from build123d import *

# Parameters (mm, degrees)
ESBO_O1_R                = 27.71344859
ESBO_O1_R_2              = 19.642943244
ESBO_O1_R_3              = 19
ESBO_O1_R_4              = 13.503376128
ESBO_O1_R_5              = 12.848056377
ESBO_O1_R_6              = 13.183675058
ESBO_O1_R_7              = 19.84940304
ESBO_O1_R_8              = 26.715530758
RESSALTO_EXTRUS_O1_DEPTH = 25


with BuildPart() as part:
    # Esboço1 → Ressalto-extrusão1 (new body)
    with BuildSketch(Plane.XY):
        with BuildLine():
            Line((4413.114192809, 5114.37123775), (4411.288420867, 5118.493395975))
            Line((4411.288420867, 5118.493395975), (4368.528056031, 5195.933053436))
            ThreePointArc((4368.528056031, 5195.933053436), (4356.563983348, 5205.481641807), (4341.352234835, 5203.77363647))
            Line((4341.352234835, 5203.77363647), (4082.380260599, 5060.775378681))
            add(Edge.make_bspline(
                [(4082.380260599, 5060.775378681), (4060.653279964, 5053.050323004), (4026.458640538, 5040.417178177), (3971.383313993, 5041.975441307), (3943.204327614, 5021.389877069), (3939.014113572, 5001.580075286)],
                knots=[0, 0, 0, 0, 0.428929879, 0.656274084, 1, 1, 1, 1], degree=3))
            ThreePointArc((3939.014113572, 5001.580075286), (3854.618299216, 4881.369865741), (3728.462541381, 4806.151033491))
            Line((3728.462541381, 4806.151033491), (3611.066608375, 4763.191643283))
            ThreePointArc((3611.066608375, 4763.191643283), (3582.494949017, 4751.209944567), (3563.519721499, 4726.718281428))
            ThreePointArc((3563.519721499, 4726.718281428), (3118.29371103, 4388.982433408), (2718.593133711, 4779.534801123))
            ThreePointArc((2718.593133711, 4779.534801123), (2705.787983512, 4805.584059889), (2678.739524891, 4816.115756812))
            Line((2678.739524891, 4816.115756812), (2629.622746024, 4816.115756812))
            ThreePointArc((2629.622746024, 4816.115756812), (2601.338474777, 4804.400028059), (2589.622746024, 4776.115756812))
            Line((2589.622746024, 4776.115756812), (2589.622746024, 4553.908462806))
            ThreePointArc((2589.622746024, 4553.908462806), (2591.760392869, 4544.912000181), (2597.716380001, 4537.838663551))
            Line((2597.716380001, 4537.838663551), (2798.624846243, 4388.982433408))
            ThreePointArc((2798.624846243, 4388.982433408), (2961.516175194, 4298.989299254), (3144.993895299, 4267.872174271))
            add(Edge.make_bspline(
                [(3144.993895299, 4267.872174271), (3283.087901646, 4272.524252265), (3410.561847837, 4324.25862746)],
                knots=[0, 0, 0, 1, 1, 1], degree=2))
            ThreePointArc((3410.561847837, 4324.25862746), (3484.943379958, 4345.587286722), (3538.443267038, 4401.491545139))
            Line((3538.443267038, 4401.491545139), (3794.487917499, 4702.904338366))
            Line((3794.487917499, 4702.904338366), (4192.149360938, 4931.885643495))
            ThreePointArc((4192.149360938, 4931.885643495), (4227.105543109, 4943.536998483), (4263.361778436, 4936.966294947))
            ThreePointArc((4263.361778436, 4936.966294947), (4268.091109103, 4934.591237745), (4272.639430224, 4931.885643495))
            ThreePointArc((4272.639430224, 4931.885643495), (4348.822764296, 4947.270554666), (4358.86043695, 5024.340918684))
            Line((4358.86043695, 5024.340918684), (4338.204141009, 5062.928165106))
            ThreePointArc((4338.204141009, 5062.928165106), (4337.44919525, 5070.544509417), (4342.300936695, 5076.463905392))
            Line((4342.300936695, 5076.463905392), (4413.114192809, 5114.37123775))
        make_face()
        with Locations((3455.392827489, 4402.582392469)):
            Circle(ESBO_O1_R, mode=Mode.SUBTRACT)
        with Locations((2639.499035595, 4588.634415219)):
            Circle(ESBO_O1_R_2, mode=Mode.SUBTRACT)
        with Locations((2639.499035595, 4726.718281428)):
            Circle(ESBO_O1_R_3, mode=Mode.SUBTRACT)
        with Locations((3582.436878638, 4633.880010415)):
            Circle(ESBO_O1_R_4, mode=Mode.SUBTRACT)
        with Locations((3643.311799709, 4690.484232349)):
            Circle(ESBO_O1_R_5, mode=Mode.SUBTRACT)
        with Locations((2639.499035595, 4776.115756812)):
            Circle(ESBO_O1_R_3, mode=Mode.SUBTRACT)
        with Locations((3701.689462413, 4743.876157041)):
            Circle(ESBO_O1_R_6, mode=Mode.SUBTRACT)
        with Locations((4005.237906418, 4932.680988887)):
            Circle(ESBO_O1_R_7, mode=Mode.SUBTRACT)
        with Locations((4299.978946887, 4992.820828576)):
            Circle(ESBO_O1_R_8, mode=Mode.SUBTRACT)
    extrude(amount=RESSALTO_EXTRUS_O1_DEPTH)


solid = part.part
Work out the finished part from the listing and answer in its coordinate system (mm). A direction names the side the tool comes from. Give positions to 0.01 mm unless a question says otherwise; leave off trailing zeros. Loops run counter-clockwise (first coordinate to the right, second up) from the corner with the lowest first, then second, coordinate; pieces in that order, holes last. Notation, with made-up numbers: (38, 1) - (62, 1) arc R15 cw to (62, 29) - close; hole circle Ø2 at (-37, -4.75). An arc over 180 degrees is marked (long way). Answer in a Markdown table with one row per item.
(1) Section A-A (y = 4852) is taken. Give the vertices of the cut face in (x, z).
Results list:
| item | result |
|---|---|
| outline | (3818.43, 0) - (4053.42, 0) - (4053.42, 25) - (3818.43, 25) - close |
(2) For a pull along Y with two mould halves and no side action, classify faces 1 (the face through (2601.65, 4804.71, 12.32)), 2 (the face through (2635.38, 4708.17, 12.32)), 3 (the face through (3990.535, 4815.792, 12.325)) as pulls with the +Y half, pulls with the -Y half, needs draft (parallel to the pull), parting line crosses it, or undercut.
Results list:
| item | result |
|---|---|
| face 1 | pulls with the +Y half |
| face 2 | undercut |
| face 3 | pulls with the -Y half |
(3) A tool of negligible diameter and unlimited length cuts with its end or side. For faces 4 (the face through (4377.21, 5095.15, 12.32)), 5 (the face through (3582.844, 4751.476, 12.325)), 6 (the face through (4312.31, 4969.12, 12.32)), from which of +Z, -Z, +X, -X, +Y, -Y can it reach the whole face along a straight path? Write none if from no direction.
Results list:
| item | result |
|---|---|
| face 4 | +Z, -Z, +X |
| face 5 | +Z, -Z, +Y |
| face 6 | +Z, -Z |
(4) Section B-B (x = 3037) is taken. Give the vertices of the cut face in (y, z).
Results list:
| item | result |
|---|---|
| outline | (4278.43, 0) - (4402, 0) - (4402, 25) - (4278.43, 25) - close |
(5) Section C-C (z = 18) is taken. State how many separate pieces and enclosed holes the cut face has, and give its area (3 significant figures).
Results list:
| item | result |
|---|---|
| separate pieces | 1 |
| enclosed holes | 9 |
| area | 328,000 mm² |
(6) Consider L1, parallel to X at y = 4573, z = 14.75; L2, parallel to X at y = 4427, z = 2.25; L3, parallel to X at y = 4922.5, z = 16. Determine where each line is inside the solid, lowest interval first. Write a range as [from, to].
Results list:
| item | result |
|---|---|
| L1 | x = [2589.62, 2627.61], [2651.39, 2792.79], [3497.2, 3684.14] |
| L2 | x = [2747.31, 2966.82], [3323.16, 3442.28], [3468.5, 3560.11] |
| L3 | x = [3892.41, 3988.2], [4022.28, 4175.85] |
(7) Flat-ended cylindrical pins translate along their axes: pin 1 Ø16 at (x, y) = (3701.69, 4743.88) entering from +Z; pin 2 Ø2 at (y, z) = (4674, 18) entering from +X; pin 3 Ø1.5 at (x, z) = (3768.5, 21) entering from -Y; pin 4 Ø1 at (x, z) = (3575, 5.5) entering from -Y. Find the tip coordinate at first contact, or state that the pin passes through.
Results list:
| item | result |
|---|---|
| pin 1 | passes through |
| pin 2 | stops at x = 3770.78 |
| pin 3 | stops at y = 4671.43 |
| pin 4 | stops at y = 4443.94 |
